Answer from the drawing. Dimensions are ordinates in mm from the lowest x, y and z of the part. A direction names the side the tool comes from. Give positions to 0.01 mm unless a question says otherwise; leave off trailing zeros. Order: outer loops, then holes, each group sorted by start corner. A loop starts at its lowest first (then second) coordinate and runs counter-clockwise, first axis right, second up. Notation, with made-up numbers: (-40, -36) -> (1, -36) arc R23 ccw to (1, 2) -> close; hole circle Ø2 at (-12, 11.5). An arc over 180 degrees is marked (long way). Write item = value, one per line. Start each with the question number.
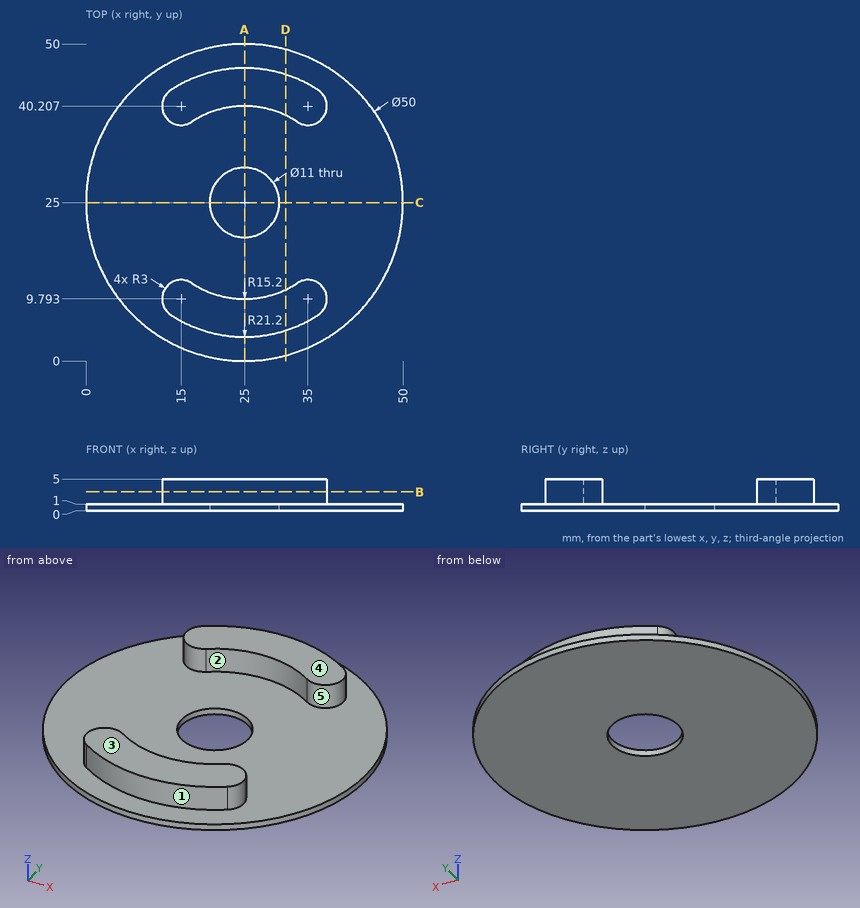
Item 1: A cutting plane is placed at B-B, the plane z = 2.95. Write down the section's boundary in (x, y), plus the area to 3 significant figures.
Item 2: Consider L1, parallel to Z at x = 6, y = 39.5; L2, parallel to Y at x = 27.5, z = 2.5; L3, parallel to Y at x = 28, z = 0.45. Determine where each line is inside the solid, lowest interval first. Write a range as from..to.
Item 3: The mould has two halves that part along X. Classify the marked faces 1, 2 and 3: +X half, -X half, draft (parallel to the pull), parting line (faces both ways), or undercut.
Item 4: A cutting plane is placed at D-D, the plane x = 31.5. Write down the section's boundary in (y, z).
Item 5: A cutting plane is placed at C-C, the plane y = 25. Write down the section's boundary in (x, z).
Item 6: A cutting plane is placed at A-A, the plane x = 25. Write down the section's boundary in (y, z).
Item 7: Flat-ended cylindrical pins translate along their axes: pin 1 (3 mm diameter, centred on x = 19, z = 3.5, fed in from +Y); pin 2 (15 mm diameter, centred on x = 27, y = 24, fed in from +Z); pin 3 (1.5 mm diameter, centred on x = 36.5, y = 16.5, fed in from -Z); pin 4 (1 mm diameter, centred on y = 8.5, z = 2, fed in from +X). Find the tip coordinate at first contact, or state that the pin passes through.
Item 8: Which of the six approach directions +Z, -Z, +X, -X, +Y, -Y give full straight-line access (tool end or side, diameter ignored) to the marked faces 4 and 5?
Check values:
q1.outline = (13.35, 7.29) arc R21.2 ccw to (36.65, 7.29) arc R3 ccw to (33.35, 12.3) arc R15.2 cw to (16.65, 12.3) arc R3 ccw to start; (13.35, 42.71) arc R3 ccw to (16.65, 37.7) arc R15.2 cw to (33.35, 37.7) arc R3 ccw to (36.65, 42.71) arc R21.2 ccw to start
q1.area = 311 mm^2
q2.L1 = 0..1
q2.L2 = 3.95..10.01, 39.99..46.05
q2.L3 = 0.18..20.39, 29.61..49.82
q3.face_1 = parting line
q3.face_2 = undercut
q3.face_3 = draft
q4.outline = (0.86, 0) -> (49.14, 0) -> (49.14, 1) -> (45.18, 1) -> (45.18, 5) -> (38.74, 5) -> (38.74, 1) -> (11.26, 1) -> (11.26, 5) -> (4.82, 5) -> (4.82, 1) -> (0.86, 1) -> close
q5.outline = (0, 0) -> (19.5, 0) -> (19.5, 1) -> (0, 1) -> close; (30.5, 0) -> (50, 0) -> (50, 1) -> (30.5, 1) -> close
q6.outline = (0, 0) -> (19.5, 0) -> (19.5, 1) -> (9.8, 1) -> (9.8, 5) -> (3.8, 5) -> (3.8, 1) -> (0, 1) -> close; (30.5, 0) -> (50, 0) -> (50, 1) -> (46.2, 1) -> (46.2, 5) -> (40.2, 5) -> (40.2, 1) -> (30.5, 1) -> close
q7.pin_1 = 45.72
q7.pin_2 = 1
q7.pin_3 = 0
q7.pin_4 = 37.89
q8.face_4 = +Z, +X, -X, +Y, -Y
q8.face_5 = +Z
